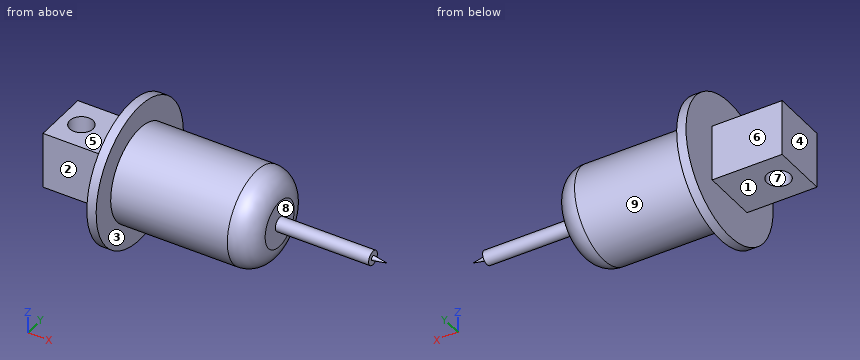
from build123d import *

# Parameters (mm, degrees)
SKETCH1_R             = 10
BOSS_EXTRUDE1_DEPTH   = 30
SKETCH4_R             = 15
BOSS_EXTRUDE2_DEPTH   = 2
FILLET1_R             = 5
SKETCH6_R             = 1.5
BOSS_EXTRUDE3_DEPTH   = 20
SKETCH7_W             = 12.06257879
SKETCH7_H             = 12
BOSS_EXTRUDE4_DEPTH   = 15
SKETCH8_R             = 2.5
CUT_EXTRUDE2_DEPTH    = 22.031289395
BODY_MOVE_COPY5_ANGLE = 90


with BuildPart() as part:
    # Sketch1 → Boss-Extrude1 (new body)
    with BuildSketch(Plane.XY):
        Circle(SKETCH1_R)
    extrude(amount=BOSS_EXTRUDE1_DEPTH)

    # Sketch4 → Boss-Extrude2 (add)
    with BuildSketch(Plane(origin=(0, 0, 0), x_dir=(-1, 0, 0), z_dir=(0, 0, -1))):
        Circle(SKETCH4_R)
    extrude(amount=BOSS_EXTRUDE2_DEPTH)

    # Fillet1
    fillet1_edges = [part.edges().sort_by_distance(p)[0] for p in [
        (-10, 0, 30),
    ]]
    fillet(fillet1_edges, radius=FILLET1_R)

    # Sketch6 → Boss-Extrude3 (add)
    with BuildSketch(Plane.XY.offset(30)):
        Circle(SKETCH6_R)
    extrude(amount=BOSS_EXTRUDE3_DEPTH)

    # Sketch7 → Boss-Extrude4 (add)
    with BuildSketch(Plane(origin=(0, 0, -2), x_dir=(-1, 0, 0), z_dir=(0, 0, -1))):
        Rectangle(SKETCH7_W, SKETCH7_H)
    extrude(amount=BOSS_EXTRUDE4_DEPTH)

    # Sketch8 → Cut-Extrude2 (cut, through all)
    with BuildSketch(Plane.ZY.offset(6.031289395)):
        with Locations((-12.5, 0)):
            Circle(SKETCH8_R)
    extrude(amount=-CUT_EXTRUDE2_DEPTH, mode=Mode.SUBTRACT)

    # Sketch15 → Revolve2 (revolve)
    with BuildSketch(Plane(origin=(0, 0, 0), x_dir=(1, 0, 0), z_dir=(0, 1, 0))):
        Polygon((0.5, -50), (0, -53), (0, -50), align=None)
    revolve(axis=Axis((0, 0, 50), (0, 0, 1)))


with BuildPart() as part_1:
    # Body-Move/Copy3: moved
    add(part.part.moved(Location((0, 0, -50))))


with BuildPart() as part_2:
    # Body-Move/Copy5: moved
    add(part_1.part.rotate(Axis((0, 0, 0), (0, 1, 0)), BODY_MOVE_COPY5_ANGLE))


solid = part_2.part
Check sheet for the modelled part. Datum: model origin and axes. Units: mm. Face numbers are marked on the shaded views. A direction names the side the tool comes from. Give positions to 0.01 mm unless a question says otherwise; leave off trailing zeros. Loops run counter-clockwise (first coordinate to the right, second up) from the corner with the lowest first, then second, coordinate; pieces in that order, holes last. Notation, with made-up numbers: M 64.5,88 L 112.5,88 A13 ccw 112.5,110 Z; hole C 21.5,42 d2. An arc over 180 degrees is marked long. Use a Markdown table: item, result. Add a question column.
Q1. Sectioned sample at A-A, the plane x = -62.5. Record the cut outline in (y, z).
Q2. Sectioned sample at C-C, the plane x = -3. Record the cut outline in (y, z), then the cut area to 3 significant figures.
Q3. Go/stop test with flat-tipped pins: pin 1 (5 mm diameter, centred on y = 7.5, z = -6.5, fed in from +X); pin 2 (6 mm diameter, centred on x = -5.5, z = 0, fed in from +Y); pin 3 (1 mm diameter, centred on y = 10, z = 0.5, fed in from -X). Record where each tip stops, or that it passes through.
Q4. Scan lines: line 1 along Y through (x, z) = (-62.5, 0.5); line 2 along X through (y, z) = (-6.75, 12.75); line 3 along Y through (x, z) = (-60.5, -5.75). Record each from-to range of solid material in increasing order. Write a range as [from, to].
Q5. Sectioned sample at B-B, the plane z = 12. Record the cut outline in (x, y).
Q6. Mould release check, pull along Y, two halves, no side actions. Record for the marked faces 6, 7, 8 and 9: pulls with the +Y half, pulls with the -Y half, needs draft (parallel to the pull), parting line crosses it, or undercut.
Q7. Tool access check on the marked faces 1, 2, 3, 4 and 5. Record the directions out of +Z, -Z, +X, -X, +Y, -Y that give a thin tool (end or side, any length) a straight path to the whole face; none if there is none.
Q8. Sectioned sample at D-D, the plane x = -30. Record the cut outline in (y, z).
Verdict:
| question | item | result |
|---|---|---|
| 1 | outline | M -6,-6.03 L -2.5,-6.03 L -2.5,6.03 L -6,6.03 Z; M 2.5,-6.03 L 6,-6.03 L 6,6.03 L 2.5,6.03 Z |
| 2 | outline | C 0,0 d3 |
| 2 | area | 7.07 mm^2 |
| 3 | pin 1 | x = -20.63 |
| 3 | pin 2 | y = 1.5 |
| 3 | pin 3 | x = -52 |
| 4 | line 1 | [-6, -2.5], [2.5, 6] |
| 4 | line 2 | [-52, -50] |
| 4 | line 3 | [-6, -1.5], [1.5, 6] |
| 5 | outline | M -52,-9 L -50,-9 L -50,9 L -52,9 Z |
| 6 | face 6 | pulls with the +Y half |
| 6 | face 7 | undercut |
| 6 | face 8 | needs draft |
| 6 | face 9 | parting line crosses it |
| 7 | face 1 | -Z, -X, +Y, -Y |
| 7 | face 2 | +Z, -Z, -X, -Y |
| 7 | face 3 | +X |
| 7 | face 4 | +Z, -Z, -X, +Y, -Y |
| 7 | face 5 | +Z, -X, +Y, -Y |
| 8 | outline | C 0,0 d20 |
